Source: CAD feature listing. Evaluate the final solid. Frame: model axes, mm. A direction names the side the tool comes from. Give positions to 0.01 mm unless a question says otherwise; leave off trailing zeros. Order: outer loops, then holes, each group sorted by start corner. A loop starts at its lowest first (then second) coordinate and runs counter-clockwise, first axis right, second up.
```python
from build123d import *

# Parameters (mm, degrees)
SKETCH_1_W          = 20.8
SKETCH_1_H          = 20.8
EXTRUDE_1_DEPTH     = 6.1
EXTRUDE_START       = -6.1
SKETCH_2_W          = 2.6
SKETCH_2_H          = 20.8
EXTRUDE_2_DEPTH     = 11.9
SKETCH_3_W          = 20.8
SKETCH_3_H          = 5.7
CUT_EXTRUDE_1_DEPTH = 2


with BuildPart() as part:
    # 草图1 → 凸台-拉伸1 (new body)
    with BuildSketch(Plane(origin=(0, 0, 0), x_dir=(1, 0, 0), z_dir=(0, 1, 0))):
        Rectangle(SKETCH_1_W, SKETCH_1_H)
    extrude(amount=EXTRUDE_1_DEPTH)

    # 草图2 → 凸台-拉伸2 (add)
    with BuildSketch(Plane(origin=(0, 6.1, 0), x_dir=(1, 0, 0), z_dir=(0, 1, 0)).offset(EXTRUDE_START)):
        with Locations((-9.1, 0)):
            Rectangle(SKETCH_2_W, SKETCH_2_H)
        with Locations((9.1, 0)):
            Rectangle(SKETCH_2_W, SKETCH_2_H)
    extrude(amount=EXTRUDE_2_DEPTH)

    # 草图3 → 切除-拉伸1 (cut)
    with BuildSketch(Plane.XZ):
        with Locations((0, -7.55)):
            Rectangle(SKETCH_3_W, SKETCH_3_H)
    extrude(amount=-CUT_EXTRUDE_1_DEPTH, mode=Mode.SUBTRACT)


solid = part.part
```
1) Section query B-B, the plane z = 2.75. Return the cut outline in (x, y).
Report:
outline: (-10.4, 0) - (10.4, 0) - (10.4, 11.9) - (7.8, 11.9) - (7.8, 6.1) - (-7.8, 6.1) - (-7.8, 11.9) - (-10.4, 11.9) - close
2) Draft query along X for faces 1 (the flat face through (10.4, 6, 0)), 2 (the flat face through (-7.8, 9, 0)), 3 (the flat face through (9, 11.9, 0)). Return one class per face: +X half, -X half, draft (parallel to the pull), parting line (faces both ways), or undercut.
Report:
face 1: +X half
face 2: undercut
face 3: draft
3) Pin query (flat end, axial travel): pin 1 (1.7 mm diameter, centred on x = 0.5, z = -8, fed in from -Y); pin 2 (5 mm diameter, centred on x = -4, z = -3, fed in from +Y). Return the tip coordinate at first contact, or that it passes through.
Report:
pin 1: stops at y = 2
pin 2: stops at y = 6.1
4) Section query D-D, the plane y = 1.5. Return the cut outline in (x, z).
Report:
outline: (-10.4, -4.7) - (10.4, -4.7) - (10.4, 10.4) - (-10.4, 10.4) - close
5) Material intervals for L1, parallel to X at y = 9, z = 0; L2, parallel to Y at x = -0.5, z = 7.5; L3, parallel to Z at x = 7, y = 1.75, sorted ascending.
Report:
L1: x = -10.4 to -7.8, 7.8 to 10.4
L2: y = 0 to 6.1
L3: z = -4.7 to 10.4
6) Reachability of faces 4 (the flat face through (0, 5, -10.4)), 5 (the flat face through (0, 1, -4.7)), 6 (the flat face through (0, 6.1, 0)) from +Z, -Z, +X, -X, +Y, -Y: full face, straight path, thin tool, end or side. Return the list, or none.
Report:
face 4: -Z, +X, -X, +Y, -Y
face 5: -Z, +X, -X, -Y
face 6: +Z, -Z, +Y
7) Section query C-C, the plane x = 9.25. Return the cut outline in (y, z).
Report:
outline: (0, -4.7) - (2, -4.7) - (2, -10.4) - (11.9, -10.4) - (11.9, 10.4) - (0, 10.4) - close
8) Section query A-A, the plane y = 10. Return the cut outline in (x, z).
Report:
outline: (-10.4, -10.4) - (-7.8, -10.4) - (-7.8, 10.4) - (-10.4, 10.4) - close; (7.8, -10.4) - (10.4, -10.4) - (10.4, 10.4) - (7.8, 10.4) - close
